Input: part model. Units: mm. Frame: model coordinates. A direction names the side the tool comes from. Give positions to 0.01 mm unless a question says otherwise; leave off trailing zeros. Loops run counter-clockwise (first coordinate to the right, second up) from the corner with the lowest first, then second, coordinate; pieces in that order, holes last.
from build123d import *

# Parameters (mm, degrees)
F0_W     = 100
F0_H     = 1.6
F1_DEPTH = 24
F2_W     = 8
F2_H     = 40
F3_DEPTH = 10
F4_W     = 8
F4_H     = 40
F5_DEPTH = 10
F6_W     = 8
F6_H     = 40
F7_DEPTH = 10
F8_W     = 10
F8_H     = 8
F9_DEPTH = 10


with BuildPart() as f1:
    # F0 (on Front) → F1 (new body, symmetric)
    with BuildSketch(Plane.XZ):
        Rectangle(F0_W, F0_H)
    extrude(amount=F1_DEPTH, both=True)

    # F2 (on face) → F3 (join)
    with BuildSketch(Plane.XY.offset(0.8)):
        with Locations((-42.821201, -2.99572)):
            Rectangle(F2_W, F2_H)
    extrude(amount=F3_DEPTH)

    # F4 (on face) → F5 (join)
    with BuildSketch(Plane.XY.offset(0.8)):
        with Locations((46, 1.605854)):
            Rectangle(F4_W, F4_H)
    extrude(amount=F5_DEPTH)

    # F6 (on face) → F7 (join)
    with BuildSketch(Plane.XY.offset(0.8)):
        with Locations((26, 1.631008)):
            Rectangle(F6_W, F6_H)
    extrude(amount=F7_DEPTH)

    # F8 (on face) → F9 (join)
    with BuildSketch(Plane.XY.offset(0.8)):
        with Locations((11.315175, -18.378249)):
            Rectangle(F8_W, F8_H)
    extrude(amount=F9_DEPTH)


solid = f1.part
(1) Mould query, pull axis X, two halves, no side actions, for faces 4 (the flat face through (-1, 0, 0.8)), 5 (the flat face through (50, 0, 5)), 6 (the flat face through (11, -18, 10.8)). Classes: +X half, -X half, draft (parallel to the pull), parting line (faces both ways), or undercut.
Values follow:
face 4: undercut
face 5: +X half
face 6: draft
(2) Cut plane D-D (x = 14). Return the cut outline in (y, z), and give its area (3 significant figures).
Values follow:
outline: (-24, -0.8) - (24, -0.8) - (24, 0.8) - (-14.38, 0.8) - (-14.38, 10.8) - (-22.38, 10.8) - (-22.38, 0.8) - (-24, 0.8) - close
area: 157 mm2
(3) Cut plane C-C (y = -12). Return the cut outline in (x, z), and give its area (3 significant figures).
Values follow:
outline: (-50, -0.8) - (50, -0.8) - (50, 10.8) - (42, 10.8) - (42, 0.8) - (30, 0.8) - (30, 10.8) - (22, 10.8) - (22, 0.8) - (-38.82, 0.8) - (-38.82, 10.8) - (-46.82, 10.8) - (-46.82, 0.8) - (-50, 0.8) - close
area: 400 mm2
(4) Ray query, probe 1 along X at (y, z) = (1, 2.5); probe 2 along X at (y, z) = (-14.5, 5.25); probe 3 along X at (y, z) = (-19, 9.5). Return the intervals inside material, ascending.
Values follow:
probe 1: x = -46.82 to -38.82, 22 to 30, 42 to 50
probe 2: x = -46.82 to -38.82, 6.32 to 16.32, 22 to 30, 42 to 50
probe 3: x = -46.82 to -38.82, 6.32 to 16.32
(5) Reachability of faces 1 (the flat face through (-43, 17.004, 6)), 2 (the flat face through (11, -14.378, 6)), 3 (the flat face through (30, 1, 6)) from +Z, -Z, +X, -X, +Y, -Y: full face, straight path, thin tool, end or side. Return the list, or none.
Values follow:
face 1: +Z, -X, +Y
face 2: +Z, +Y
face 3: +Z, +Y, -Y
(6) Pin query (flat end, axial travel): pin 1 Ø6.5 at (y, z) = (-19, 3.5) entering from +X; pin 2 Ø3 at (x, z) = (10, 4.5) entering from +Y; pin 3 Ø4 at (x, y) = (15.5, 16) entering from +Z; pin 4 Ø6.5 at (x, z) = (28, 6.5) entering from +Y. Return the tip coordinate at first contact, or that it passes through.
Values follow:
pin 1: stops at x = 50
pin 2: stops at y = -14.38
pin 3: stops at z = 0.8
pin 4: stops at y = 21.63
(7) Cut plane A-A (z = 7.5). Return the cut outline in (x, y), and give its area (3 significant figures).
Values follow:
outline: (-46.82, -23) - (-38.82, -23) - (-38.82, 17) - (-46.82, 17) - close; (6.32, -22.38) - (16.32, -22.38) - (16.32, -14.38) - (6.32, -14.38) - close; (22, -18.37) - (30, -18.37) - (30, 21.63) - (22, 21.63) - close; (42, -18.39) - (50, -18.39) - (50, 21.61) - (42, 21.61) - close
area: 1,040 mm2
(8) Cut plane B-B (x = -41). Return the cut outline in (y, z), and give its area (3 significant figures).
Values follow:
outline: (-24, -0.8) - (24, -0.8) - (24, 0.8) - (17, 0.8) - (17, 10.8) - (-23, 10.8) - (-23, 0.8) - (-24, 0.8) - close
area: 477 mm2
